Can you work these out from the model? Positions are in its coordinate system, mm. Face numbers are marked on the shaded views. A direction names the side the tool comes from. Give positions to 0.01 mm unless a question says otherwise; leave off trailing zeros. Write each loop counter-clockwise with the first axis right and the second up, starting at its lowest first coordinate (ties: lowest second). Pieces come first, ordered by that corner, then holes.
1. Suppose I cut it at C-C (z = 3.5). Give the number of separate pieces and of enclosed holes in the cut face, and give its area (3 significant figures).
2. Suppose I cut it at B-B (y = -12). Please give me the cut outline in (x, z), and give its area (3 significant figures).
3. On a 3-axis mill with a long thin cutter (end or side, diameter ignored), from which of +Z, -Z, +X, -X, +Y, -Y can I reach the whole of each face in a straight line? I mean the marked faces 1 and 2. Say none if no direction works.
4. If I drill on probe 1 along X at (y, z) = (-25, 3); probe 2 along Y at (x, z) = (10.2, 6.5) (3 decimals); probe 3 along Z at (x, y) = (6, 3.5), over which ranges is the centre line in solid material (lowest first)?
5. I'm going to push flat-ended pins straight in: pin 1 (4 mm diameter, centred on y = -24, z = 7, fed in from +X); pin 2 (4 mm diameter, centred on y = -24.5, z = 6, fed in from -X); pin 3 (6.5 mm diameter, centred on y = 17.5, z = 8, fed in from -X). Where does each tip first touch, or does it pass through?
6. Suppose I cut it at A-A (x = 0). Please give me the cut outline in (y, z) (3 decimals).
7. Suppose I cut it at D-D (y = 10). Please give me the cut outline in (x, z).
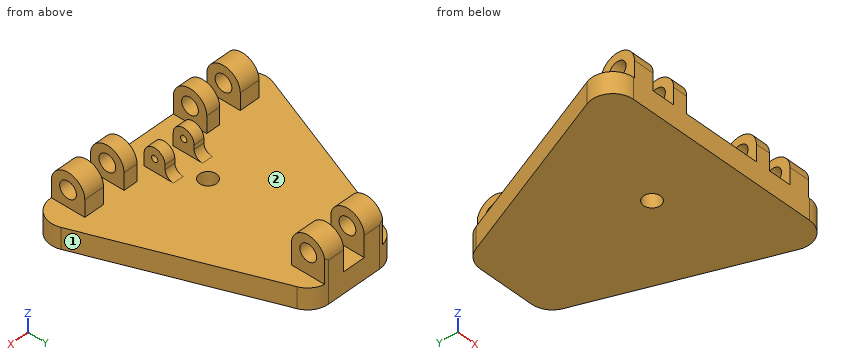
```python
from build123d import *

# Parameters (mm, degrees)
BOSS_EXTRUDE1_DEPTH = 2.5
SKETCH2_R           = 2
BOSS_EXTRUDE2_DEPTH = 22.5
CUT_EXTRUDE1_REACH  = 62.519
SKETCH3_W           = 18
SKETCH3_H           = 16
SKETCH3_W_2         = 5.3
SKETCH7_R           = 2
BOSS_EXTRUDE4_DEPTH = 7.5
SKETCH8_W           = 5.3
SKETCH8_H           = 18
CUT_EXTRUDE4_DEPTH  = 8
SKETCH4_R           = 0.75
BOSS_EXTRUDE3_DEPTH = 5
SKETCH5_W           = 5
SKETCH5_H           = 11
CUT_EXTRUDE2_DEPTH  = 52.696228102
FILLET2_R           = 2
SKETCH6_R           = 2
CUT_EXTRUDE3_DEPTH  = 43.431010181
FILLET4_R           = 5


with BuildPart() as part:
    # Sketch1 → Boss-Extrude1 (new, symmetric)
    with BuildSketch(Plane.XY):
        Polygon((-30, -28.625), (30, -28.625), (10, 22.875), (-10, 22.875), align=None)
    extrude(amount=BOSS_EXTRUDE1_DEPTH, both=True)

    # Sketch2 → Boss-Extrude2 (add, symmetric)
    with BuildSketch(Plane(origin=(0, 0, 0), x_dir=(0, 0, -1), z_dir=(1, 0, 0))):
        with BuildLine():
            Line((-2.5, -28.625), (-6.5, -28.625))
            ThreePointArc((-6.5, -28.625), (-10.5, -24.625), (-6.5, -20.625))
            Line((-6.5, -20.625), (-2.5, -20.625))
            Line((-2.5, -20.625), (-2.5, -28.625))
        make_face()
        with Locations(Location((-6.5, -24.625, 0), (0, 0, 180))):
            Circle(SKETCH2_R, mode=Mode.SUBTRACT)
    extrude(amount=BOSS_EXTRUDE2_DEPTH, both=True)

    # Sketch3 → Cut-Extrude1 (cut, up to next)
    with BuildSketch(Plane.XZ.offset(28.625), mode=Mode.PRIVATE) as cut_extrude1_sk1:
        with Locations((0, 10.5)):
            Rectangle(SKETCH3_W, SKETCH3_H)
    cut_extrude1_tool1 = extrude(cut_extrude1_sk1.sketch, amount=-CUT_EXTRUDE1_REACH, mode=Mode.PRIVATE) & part.part
    # Sketch3 → Cut-Extrude1 (cut, up to next)
    with BuildSketch(Plane.XZ.offset(28.625), mode=Mode.PRIVATE) as cut_extrude1_sk2:
        with Locations((-15, 10.5)):
            Rectangle(SKETCH3_W_2, SKETCH3_H)
    cut_extrude1_tool2 = extrude(cut_extrude1_sk2.sketch, amount=-CUT_EXTRUDE1_REACH, mode=Mode.PRIVATE) & part.part
    cut_extrude1_1 = cut_extrude1_tool1.solids().sort_by_distance((0, -28.625, 10.5))[0]
    add(cut_extrude1_1, mode=Mode.SUBTRACT)
    cut_extrude1_2 = cut_extrude1_tool2.solids().sort_by_distance((-15, -28.625, 10.5))[0]
    add(cut_extrude1_2, mode=Mode.SUBTRACT)
    cut_extrude1 = cut_extrude1_1 + cut_extrude1_2  # Cut-Extrude1 as one shape, for the pattern or mirror that repeats it

    # Mirror2: Cut-Extrude1 across plane
    add(cut_extrude1.mirror(Plane(origin=(0, 0, 0), x_dir=(0, 0, 1), z_dir=(1, 0, 0))), mode=Mode.SUBTRACT)

    # Sketch7 → Boss-Extrude4 (add, symmetric)
    with BuildSketch(Plane(origin=(0, 0, 0), x_dir=(0, 0, -1), z_dir=(1, 0, 0))):
        with BuildLine():
            Line((-2.5, 14.875), (-7.5, 14.875))
            ThreePointArc((-7.5, 14.875), (-11.5, 18.875), (-7.5, 22.875))
            Line((-7.5, 22.875), (-2.5, 22.875))
            Line((-2.5, 22.875), (-2.5, 14.875))
        make_face()
        with Locations((-7.5, 18.875)):
            Circle(SKETCH7_R, mode=Mode.SUBTRACT)
    extrude(amount=BOSS_EXTRUDE4_DEPTH, both=True)

    # Sketch8 → Cut-Extrude4 (cut)
    with BuildSketch(Plane(origin=(0, 22.875, 0), x_dir=(1, 0, 0), z_dir=(0, 1, 0))):
        with Locations((0, -11.5)):
            Rectangle(SKETCH8_W, SKETCH8_H)
    extrude(amount=-CUT_EXTRUDE4_DEPTH, mode=Mode.SUBTRACT)

    # Sketch4 → Boss-Extrude3 (add, symmetric)
    with BuildSketch(Plane(origin=(0, 0, 0), x_dir=(0, 0, -1), z_dir=(1, 0, 0))):
        with BuildLine():
            Line((-2.5, -22.625), (-5.5, -22.625))
            ThreePointArc((-5.5, -22.625), (-8, -20.125), (-5.5, -17.625))
            Line((-5.5, -17.625), (-2.5, -17.625))
            Line((-2.5, -17.625), (-2.5, -22.625))
        make_face()
        with Locations((-5.5, -20.125)):
            Circle(SKETCH4_R, mode=Mode.SUBTRACT)
    extrude(amount=BOSS_EXTRUDE3_DEPTH, both=True)

    # Sketch5 → Cut-Extrude2 (cut, through all)
    with BuildSketch(Plane(origin=(0, -17.625, 0), x_dir=(1, 0, 0), z_dir=(0, 1, 0))):
        with Locations((0, -8)):
            Rectangle(SKETCH5_W, SKETCH5_H)
    extrude(amount=-CUT_EXTRUDE2_DEPTH, mode=Mode.SUBTRACT)

    # Fillet2
    fillet2_edges = [part.edges().sort_by_distance(p)[0] for p in [
        (3.75, -17.625, 2.5),
        (-3.75, -17.625, 2.5),
    ]]
    fillet(fillet2_edges, radius=FILLET2_R)

    # Sketch6 → Cut-Extrude3 (cut, through all)
    with BuildSketch(Plane.XY.offset(2.5)):
        with Locations((0, -12)):
            Circle(SKETCH6_R)
    extrude(amount=-CUT_EXTRUDE3_DEPTH, mode=Mode.SUBTRACT)

    # Fillet4
    # the kernel refuses this fillet: 5 mm, written as the material it takes off along each edge
    with BuildSketch(Plane(origin=(30, -28.625, -20.763876668), x_dir=(-1, 0, 0), z_dir=(0, 0, 1)), Plane(origin=(-30, -28.625, 20.763876668), x_dir=(1, 0, 0), z_dir=(0, 0, -1))) as fillet4_piece_1:
        with BuildLine():
            CenterArc((FILLET4_R * 1.46111013346, -FILLET4_R), FILLET4_R, 90, 111.223656503)
            Line((FILLET4_R * 0.52893572066, -FILLET4_R * 1.3620094807), (0, 0))
            Line((0, 0), (FILLET4_R * 1.46111013346, 0))
        make_face()
    extrude(amount=41.527753337, mode=Mode.SUBTRACT)
    with BuildSketch(Plane(origin=(10, 22.875, -11.055138804), x_dir=(0.3620094806999332, -0.9321744128023278, 0), z_dir=(0, 0, 1))) as fillet4_piece_2:
        with BuildLine():
            CenterArc((FILLET4_R * 0.684411104336, -FILLET4_R), FILLET4_R, 90, 68.776343497)
            Line((-FILLET4_R * 0.247763308466, -FILLET4_R * 0.6379905193), (0, 0))
            Line((0, 0), (FILLET4_R * 0.684411104336, 0))
        make_face()
    extrude(amount=22.110277608, mode=Mode.SUBTRACT)
    with BuildSketch(Plane(origin=(-10, 22.875, 11.055138804), x_dir=(1, 0, 0), z_dir=(0, 0, -1))) as fillet4_piece_3:
        with BuildLine():
            CenterArc((FILLET4_R * 0.684411104336, FILLET4_R), FILLET4_R, 201.223656503, 68.776343497)
            Line((-FILLET4_R * 0.247763308466, FILLET4_R * 0.6379905193), (0, 0))
            Line((0, 0), (FILLET4_R * 0.684411104336, 0))
        make_face()
    extrude(amount=22.110277608, mode=Mode.SUBTRACT)


solid = part.part
```
Checks:
1. separate pieces: 8
1. enclosed holes: 0
1. area: 235 mm2
2. outline: (-23.54, -2.5) - (-2, -2.5) - (-2, 2.5) - (-23.54, 2.5) - close; (2, -2.5) - (23.54, -2.5) - (23.54, 2.5) - (2, 2.5) - close
2. area: 215 mm2
3. face 1: +Z, -Z, +X, +Y
3. face 2: +Z
4. probe 1: x = -22.5 to -17.65, -12.35 to -9, 9 to 12.35, 17.65 to 22.5
4. probe 2: y = -28.625 to -26.625, -22.625 to -20.625
4. probe 3: z = -2.5 to 2.5
5. pin 1: stops at x = 22.5
5. pin 2: stops at x = -22.5
5. pin 3: stops at x = -7.5
6. outline: (-28.625, -2.5) - (-14, -2.5) - (-14, 2.5) - (-28.625, 2.5) - close; (-10, -2.5) - (22.875, -2.5) - (22.875, 2.5) - (-10, 2.5) - close
7. outline: (-15, -2.5) - (15, -2.5) - (15, 2.5) - (-15, 2.5) - close
